from build123d import *

# Parameters (mm, degrees)
SKETCH1_W               = 15
SKETCH1_H               = 80
BOSS_EXTRUDE1_DEPTH     = 75
SKETCH1_3_R             = 12.5
BOSS_EXTRUDE2_DEPTH     = 15
SKETCH1_4_R             = 12.5
SKETCH1_4_R_2           = 6
BOSS_EXTRUDE3_DEPTH     = 10
CUT_EXTRUDE1_DEPTH      = 160.530561335
CUT_EXTRUDE1_DEPTH_BACK = 160.530561335
SKETCH2_R               = 7.5


with BuildPart() as part:
    # Sketch1 → Boss-Extrude1 (new body)
    with BuildSketch(Plane(origin=(0, 0, 0), x_dir=(1, 0, 0), z_dir=(0, 1, 0))):
        with Locations((7.5, 0)):
            Rectangle(SKETCH1_W, SKETCH1_H)
    extrude(amount=BOSS_EXTRUDE1_DEPTH)

    # Sketch1_3 → Boss-Extrude2 (add)
    with BuildSketch(Plane(origin=(0, 0, 0), x_dir=(1, 0, 0), z_dir=(0, 1, 0))):
        with BuildLine():
            ThreePointArc((142.97865308, -31.684424019), (137.665581407, -37.744432147), (129.928343994, -40))
            Line((129.928343994, -40), (15, -40))
            Line((15, -40), (15, 40))
            Line((15, 40), (129.928343994, 40))
            ThreePointArc((129.928343994, 40), (137.665581407, 37.744432147), (142.97865308, 31.684424019))
            ThreePointArc((142.97865308, 31.684424019), (150, 0), (142.97865308, -31.684424019))
        make_face()
        with Locations(Location((75, 0, 0), (0, 0, 270))):
            Circle(SKETCH1_3_R, mode=Mode.SUBTRACT)
        with BuildLine():
            ThreePointArc((125.229473419, 29), (114.301270189, 31.92820323), (111.373066959, 21))
            ThreePointArc((111.373066959, 21), (117, 0), (111.373066959, -21))
            ThreePointArc((111.373066959, -21), (114.301270189, -31.92820323), (125.229473419, -29))
            ThreePointArc((125.229473419, -29), (133, 0), (125.229473419, 29))
        make_face(mode=Mode.SUBTRACT)
    extrude(amount=BOSS_EXTRUDE2_DEPTH)

    # Sketch1_4 → Boss-Extrude3 (add)
    with BuildSketch(Plane(origin=(0, 0, 0), x_dir=(1, 0, 0), z_dir=(0, 1, 0))):
        with Locations(Location((75, 0, 0), (0, 0, 270))):
            Circle(SKETCH1_4_R)
        with Locations(Location((75, 0, 0), (0, 0, 270))):
            Circle(SKETCH1_4_R_2, mode=Mode.SUBTRACT)
    extrude(amount=BOSS_EXTRUDE3_DEPTH)

    # Sketch2 → Cut-Extrude1 (cut, two sides: drawn at the far end of the back side and taken through both)
    with BuildSketch(Plane(origin=(15, 0, 0), x_dir=(0, 0, -1), z_dir=(1, 0, 0)).offset(-CUT_EXTRUDE1_DEPTH_BACK)):
        with BuildLine():
            ThreePointArc((20, 75), (34.142135624, 69.142135624), (40, 55))
            Line((40, 55), (40, 75))
            Line((40, 75), (20, 75))
        make_face()
        with Locations((20, 55)):
            Circle(SKETCH2_R)
        with Locations((-20, 55)):
            Circle(SKETCH2_R)
        with BuildLine():
            ThreePointArc((-40, 55), (-34.142135624, 69.142135624), (-20, 75))
            Line((-20, 75), (-40, 75))
            Line((-40, 75), (-40, 55))
        make_face()
    extrude(amount=CUT_EXTRUDE1_DEPTH + CUT_EXTRUDE1_DEPTH_BACK, mode=Mode.SUBTRACT)


solid = part.part
Work out the finished part from the listing and answer in its coordinate system (mm). A direction names the side the tool comes from. Give positions to 0.01 mm unless a question says otherwise; leave off trailing zeros. Order: outer loops, then holes, each group sorted by start corner. A loop starts at its lowest first (then second) coordinate and runs counter-clockwise, first axis right, second up. Notation, with made-up numbers: (-35.5, 41) - (8.5, 41) arc R26 cw to (8.5, 80) - close; hole circle Ø6 at (0, 14.5). An arc over 180 degrees is marked (long way). Answer as CSV lines item,"result". Start each with the question number.
Q1. Find the intervals of material crossed by L1, parallel to Z at x = 7, y = 55; L2, parallel to X at y = 11.5, z = -11.5; L3, parallel to X at y = 28.5, z = 31.5, in increasing order. Write a range as [from, to].
Q2. The part is cut by section C-C (y = 49). Write down the section's boundary in (x, z), then the cut area to 3 significant figures.
Q3. Given pin 1 Ø4 at (x, z) = (69, -20) entering from -Y; pin 2 Ø1.5 at (y, z) = (23, -25.5) entering from +X; pin 3 Ø12 at (x, z) = (69.5, 23.5) entering from +Y; pin 4 Ø12.5 at (x, z) = (71.5, 2) entering from +Y, each flat-ended and moving along its own axis, determine where each tip first touches the part or whether it passes through.
Q4. The part is cut by section A-A (x = 75). Write down the section's boundary in (y, z).
Q5. For faces 4 (the face through (83.44, 15, -9.45)), 5 (the face through (117, 7, 0)), 6 (the face through (87.394, 12.465, -1.627)), determine the directions among +Z, -Z, +X, -X, +Y, -Y from which every point of the face is accessible in a straight line to the end or side of a thin tool.
Q6. The part is cut by section D-D (y = 12). Write down the section's boundary in (x, z), then the cut area to 3 significant figures.
Q7. The part is cut by section B-B (z = 0). Write down the section's boundary in (x, y).
Q8. The mould has two halves that part along Z. Classify faces 1 (the face through (137.762, 7.395, 37.683)), 2 (the face through (69.6, 10, -3)), 3 (the face through (7.395, 69.297, -33.986)): +Z half, -Z half, draft (parallel to the pull), parting line (faces both ways), or undercut.
Check result:
1,L1,"z = [-40, -27.5], [-12.5, 12.5], [27.5, 40]"
1,L2,"x = [0, 70.1], [79.9, 115.39], [131.85, 149.11]"
1,L3,"x = [0, 15]"
2,outline,"(0, -40) - (15, -40) - (15, -24.5) - (0, -24.5) - close; (0, -15.5) - (15, -15.5) - (15, 15.5) - (0, 15.5) - close; (0, 24.5) - (15, 24.5) - (15, 40) - (0, 40) - close"
2,area,"930 mm²"
3,pin 1,"stops at y = 0"
3,pin 2,"stops at x = 15"
3,pin 3,"stops at y = 15"
3,pin 4,"stops at y = 10"
4,outline,"(0, -40) - (15, -40) - (15, -12.5) - (10, -12.5) - (10, -6) - (0, -6) - close; (0, 6) - (10, 6) - (10, 12.5) - (15, 12.5) - (15, 40) - (0, 40) - close"
5,face 4,"+Z, -Z, +X, +Y"
5,face 5,"+Y, -Y"
5,face 6,"+Y"
6,outline,"(0, -40) - (129.93, -40) arc R14.4 ccw to (142.98, -31.68) arc R75 ccw to (142.98, 31.68) arc R14.4 ccw to (129.93, 40) - (0, 40) - close; hole circle Ø25 at (75, 0); hole (111.37, -21) arc R8 ccw to (125.23, -29) arc R58 ccw to (125.23, 29) arc R8 ccw to (111.37, 21) arc R42 cw to start"
6,area,"10,100 mm²"
7,outline,"(0, 0) - (69, 0) - (69, 10) - (62.5, 10) - (62.5, 15) - (15, 15) - (15, 75) - (0, 75) - close; (81, 0) - (117, 0) - (117, 15) - (87.5, 15) - (87.5, 10) - (81, 10) - close; (133, 0) - (150, 0) - (150, 15) - (133, 15) - close"
8,face 1,"+Z half"
8,face 2,"undercut"
8,face 3,"-Z half"
